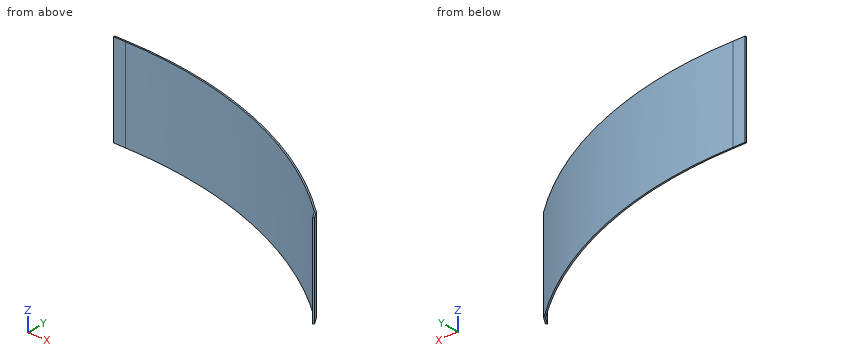
Autodesk Inventor part; units mm, degrees
ref_plane "YZ Plane" through (0, 0, 0) normal (1, 0, 0) x (0, 1, 0)
ref_plane "XZ Plane" through (0, 0, 0) normal (0, 1, 0) x (-1, 0, 0)
ref_plane "XY Plane" through (0, 0, 0) normal (0, 0, 1) x (1, 0, 0)
sketch "Sketch1" plane through (0, 0, 0) normal (0, 0, 1) x (1, 0, 0)
  line L0 (6.4002, -1.3978) -> (19.527, -1.3978)
  line L1 (6.4002, -1.3978) -> (6.4002, -2.9853)
  line L2 (6.4002, -2.9853) -> (19.527, -2.9853)
  line L3 (333.1851, -123.7146) -> (327.4784, -114.9672)
  line L4 (333.1851, -123.7146) -> (331.8555, -124.582)
  line L5 (331.8555, -124.582) -> (326.1488, -115.8346)
  arc A0 (327.4784, -114.9672) -> (19.527, -1.3978) centre (26.9726, -455.509) ccw
  arc A1 (326.1488, -115.8346) -> (19.527, -2.9853) centre (26.4701, -457.1045) ccw
  point P0 (0, 0)
  dimension "d1" = 1.5875
  dimension "d2" = 1.5875
  dimension "d3" = 454.1723
extrude "Extrusion1" add sketch "Sketch1" against normal blind 101.6
properties part number "Hood Lexan" material "Polycarbonate, Clear"
The model under review builds one solid part; all positions refer to its coordinate system, in mm. Give positions to 0.01 mm unless a question says otherwise; leave off trailing zeros. Write each loop counter-clockwise with the first axis right and the second up, starting at its lowest first coordinate (ties: lowest second). Pieces come first, ordered by that corner, then holes. Notation, with made-up numbers: (12, -0.5) -> (56, -0.5) arc R23 ccw to (56, 29.5) -> close; hole circle Ø4 at (88, 40.5). An arc over 180 degrees is marked (long way). Answer in a Markdown table with one row per item.
1) Clearance check with flat-ended pins moving along their axes: P1, Ø2, axis at y = -50, z = -16, coming from the +X side; P2, Ø6, axis at x = 140, z = -12, coming from the -Y side; P3, Ø1.5, axis at y = -55, z = -91, coming from the +X side. State where each tip first meets the part, or that it passes through.
Worked answers:
| item | result |
|---|---|
| P1 | x = 233.48 |
| P2 | y = -18.14 |
| P3 | x = 242.53 |
2) Add section C-C on x = 31. State the section outline as (y, z) points.
Worked answers:
| item | result |
|---|---|
| outline | (-2.95, -101.6) -> (-1.35, -101.6) -> (-1.35, 0) -> (-2.95, 0) -> close |
3) For L1, parallel to Y at x = 75, z = -84.5; L2, parallel to Y at x = 262, z = -50; L3, parallel to X at y = -78, z = -31, list the stretches that pass through material, from the lowest coordinate up. Write a range as [from, to].
Worked answers:
| item | result |
|---|---|
| L1 | [-5.53, -3.88] |
| L2 | [-68.78, -66.88] |
| L3 | [276.57, 279.48] |
4) Add section A-A on z = -8. State the section outline as (x, y) points, plus the area to 3 significant figures.
Worked answers:
| item | result |
|---|---|
| outline | (6.4, -2.99) -> (19.53, -2.99) arc R454.17 cw to (326.15, -115.83) -> (331.86, -124.58) -> (333.19, -123.71) -> (327.48, -114.97) arc R454.17 ccw to (19.53, -1.4) -> (6.4, -1.4) -> close |
| area | 585 mm² |
